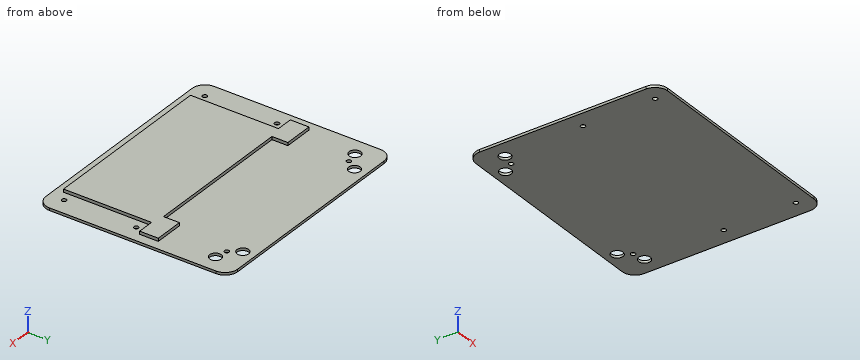
from build123d import *

# Parameters (mm, degrees)
F0_W     = 138.111218
F0_H     = 115.343272
F0_R     = 1.382409
F0_R_2   = 3.496557
F1_DEPTH = 1.524
F3_DEPTH = 1.8288
F4_R     = 7.62


with BuildPart() as f1:
    # F0 (on Top) → F1 (new body)
    with BuildSketch(Plane.XY):
        Rectangle(F0_W, F0_H)
        with Locations((-59.067786, -48.435853)):
            Circle(F0_R, mode=Mode.SUBTRACT)
        with Locations((-59.067786, -5.047345)):
            Circle(F0_R, mode=Mode.SUBTRACT)
        with Locations((59.067786, -48.435853)):
            Circle(F0_R, mode=Mode.SUBTRACT)
        with Locations((59.067786, -5.047345)):
            Circle(F0_R, mode=Mode.SUBTRACT)
        with Locations((-58.543, 42.207982)):
            Circle(F0_R_2, mode=Mode.SUBTRACT)
        with Locations((-51.227979, 43.833543)):
            Circle(F0_R, mode=Mode.SUBTRACT)
        with Locations((-46.893153, 50.335784)):
            Circle(F0_R_2, mode=Mode.SUBTRACT)
        with Locations((58.543, 42.207982)):
            Circle(F0_R_2, mode=Mode.SUBTRACT)
        with Locations((51.227979, 43.833543)):
            Circle(F0_R, mode=Mode.SUBTRACT)
        with Locations((46.893153, 50.335784)):
            Circle(F0_R_2, mode=Mode.SUBTRACT)
    extrude(amount=F1_DEPTH)

    # F2 (on face) → F3 (join)
    with BuildSketch(Plane.XY.offset(1.524)):
        Polygon((-53.286642, -52.906867), (0, -52.906867), (53.286642, -52.906867), (53.286642, 0), (63.22062, 0), (63.22062, 11.212443), (45.520075, 11.212443), (45.520075, 1.639701), (0, 1.639701), (-45.520075, 1.639701), (-45.520075, 11.212443), (-63.22062, 11.212443), (-63.22062, 0), (-53.286642, 0), align=None)
    extrude(amount=F3_DEPTH)

    # F4
    f4_edges = [f1.edges().sort_by_distance(p)[0] for p in [
        (-69.055609, 57.671636, 0.762),
        (69.055609, 57.671636, 0.762),
        (69.055609, -57.671636, 0.762),
        (-69.055609, -57.671636, 0.762),
    ]]
    fillet(f4_edges, radius=F4_R)


solid = f1.part
Geometry check sheet. Reference: the model listing, model coordinates, mm. Round coordinates to 2 decimals unless told otherwise and drop trailing zeros. Order: outer loops, then holes, each group sorted by start corner. A loop starts at its lowest first (then second) coordinate and runs counter-clockwise, first axis right, second up. Notation, with made-up numbers: M 0.5,-4.75 L 30.5,-4.75 A19 cw 30.5,31.25 Z; hole C 4,-16 d6. An arc over 180 degrees is marked long. Answer in a Markdown table with one row per item.
(1) Sectioned sample at D-D, the plane y = 13. Record the cut outline in (x, z), and give its area (3 significant figures).
Responses:
| item | result |
|---|---|
| outline | M -69.06,0 L 69.06,0 L 69.06,1.52 L -69.06,1.52 Z |
| area | 210 mm² |
(2) Sectioned sample at C-C, the plane z = 2.7. Record the cut outline in (x, y).
Responses:
| item | result |
|---|---|
| outline | M -63.22,0 L -53.29,0 L -53.29,-52.91 L 53.29,-52.91 L 53.29,0 L 63.22,0 L 63.22,11.21 L 45.52,11.21 L 45.52,1.64 L -45.52,1.64 L -45.52,11.21 L -63.22,11.21 Z |
(3) Sectioned sample at A-A, the plane x = -30.5. Record the cut outline in (y, z).
Responses:
| item | result |
|---|---|
| outline | M -57.67,0 L 57.67,0 L 57.67,1.52 L 1.64,1.52 L 1.64,3.35 L -52.91,3.35 L -52.91,1.52 L -57.67,1.52 Z |
(4) Sectioned sample at B-B, the plane y = -13.5. Record the cut outline in (x, z).
Responses:
| item | result |
|---|---|
| outline | M -69.06,0 L 69.06,0 L 69.06,1.52 L 53.29,1.52 L 53.29,3.35 L -53.29,3.35 L -53.29,1.52 L -69.06,1.52 Z |
(5) Scan lines: probe 1 along X at (y, z) = (42, 0.85); probe 2 along X at (y, z) = (47.5, 0.8); probe 3 along X at (y, z) = (6, 2.8). Record each from-to range of solid material in increasing order. Write a range as from..to.
Responses:
| item | result |
|---|---|
| probe 1 | x = -69.06..-62.03, -55.05..55.05, 62.03..69.06 |
| probe 2 | x = -69.06..-48.94, -44.85..44.85, 48.94..69.06 |
| probe 3 | x = -63.22..-45.52, 45.52..63.22 |
(6) Go/stop test with flat-tipped pins: P1, Ø1.5, axis at x = 59, z = 3, coming from the -Y side; P2, Ø0.9, axis at y = -22, z = 2.5, coming from the +X side; P3, Ø1.7, axis at x = -59.07, y = -48.44, coming from the +Z side; P4, Ø5, axis at x = 16.5, y = 45, coming from the +Z side. Record where each tip stops, or that it passes through.
Responses:
| item | result |
|---|---|
| P1 | stops at y = 0 |
| P2 | stops at x = 53.29 |
| P3 | passes through |
| P4 | stops at z = 1.52 |
